```python
from build123d import *

# Parameters (mm, degrees)
SKETCH2_R           = 6
BOSS_EXTRUDE2_DEPTH = 70
CUT_EXTRUDE1_DEPTH  = 21.875
CUT_EXTRUDE3_START  = -21.875
CUT_EXTRUDE3_DEPTH  = 21.875
SKETCH4_R           = 4.215
CUT_EXTRUDE4_DEPTH  = 72.470273541


with BuildPart() as part:
    # Sketch2 → Boss-Extrude2 (new body)
    with BuildSketch(Plane.XY):
        with BuildLine():
            ThreePointArc((-6, 0), (0, 6), (6, 0))
            Line((6, 0), (6, 5.291502622))
            ThreePointArc((6, 5.291502622), (0, 8), (-6, 5.291502622))
            Line((-6, 5.291502622), (-6, 0))
        make_face()
        Circle(SKETCH2_R)
        with BuildLine():
            Line((6, -5.291502622), (6, 0))
            ThreePointArc((6, 0), (0, -6), (-6, 0))
            Line((-6, 0), (-6, -5.291502622))
            ThreePointArc((-6, -5.291502622), (0, -8), (6, -5.291502622))
        make_face()
    extrude(amount=-BOSS_EXTRUDE2_DEPTH)

    # Sketch5 → Cut-Extrude1 (cut)
    with BuildSketch(Plane.XY):
        with BuildLine():
            ThreePointArc((6, 5.291502622), (0, 8), (-6, 5.291502622))
            Line((-6, 5.291502622), (-6, -5e-09))
            ThreePointArc((-6, -5e-09), (-2e-09, 6), (6, 0))
            Line((6, 0), (6, 5.291502622))
        make_face()
        with BuildLine():
            ThreePointArc((6, 0), (2e-09, -6), (-6, -5e-09))
            Line((-6, -5e-09), (-6, -5.291502622))
            ThreePointArc((-6, -5.291502622), (0, -8), (6, -5.291502622))
            Line((6, -5.291502622), (6, 0))
        make_face()
    extrude(amount=-CUT_EXTRUDE1_DEPTH, mode=Mode.SUBTRACT)

    # Sketch6 → Cut-Extrude3 (cut)
    with BuildSketch(Plane(origin=(0, 0, -70), x_dir=(-1, 0, 0), z_dir=(0, 0, -1)).offset(CUT_EXTRUDE3_START)):
        with BuildLine():
            ThreePointArc((6, 5.291502622), (0, 8), (-6, 5.291502622))
            Line((-6, 5.291502622), (-6, -5e-09))
            ThreePointArc((-6, -5e-09), (-2e-09, 6), (6, 0))
            Line((6, 0), (6, 5.291502622))
        make_face()
        with BuildLine():
            ThreePointArc((6, 0), (2e-09, -6), (-6, -5e-09))
            Line((-6, -5e-09), (-6, -5.291502622))
            ThreePointArc((-6, -5.291502622), (0, -8), (6, -5.291502622))
            Line((6, -5.291502622), (6, 0))
        make_face()
    extrude(amount=CUT_EXTRUDE3_DEPTH, mode=Mode.SUBTRACT)

    # Sketch4 → Cut-Extrude4 (cut, through all)
    with BuildSketch(Plane(origin=(6, 0, 0), x_dir=(0, 0, -1), z_dir=(1, 0, 0))):
        with Locations((35, 0)):
            Circle(SKETCH4_R)
    extrude(amount=-CUT_EXTRUDE4_DEPTH, mode=Mode.SUBTRACT)


solid = part.part
```
Input: part model. Units: mm. Frame: model coordinates. A direction names the side the tool comes from. Coordinates: 2 decimals unless noted, no trailing zeros. Write each loop counter-clockwise with the first axis right and the second up, starting at its lowest first coordinate (ties: lowest second). Pieces come first, ordered by that corner, then holes.
1) Pin query (flat end, axial travel): pin 1 Ø5 at (x, z) = (3, -48.5) entering from -Y; pin 2 Ø7.5 at (y, z) = (0, -35) entering from +X; pin 3 Ø1 at (y, z) = (-2.5, -13) entering from +X. Return the tip coordinate at first contact, or that it passes through.
2) Set-up query: faces 1 (the flat face through (0.4, -6.4, -21.875)), 2 (the cylindrical face through (4.76, 3.65, -58.91)), 3 (the flat face through (-0.4, 6.4, -48.125)), 4 (the flat face through (-0.4, -6.4, -48.125)). Return all of +Z, -Z, +X, -X, +Y, -Y with unobstructed straight access to the full face (end or side cutting, diameter ignored); none if empty.
3) Section B-B on x = 0. Output: boundary loops of the cut face in (y, z) (3 decimals).
4) Section A-A on z = -35. Output: boundary loops of the cut face in (x, y) (1 decimal).
5) Section D-D on z = -65. Output: boundary loops of the cut face in (x, y), and give its area (3 significant figures).
6) Mould query, pull axis Y, two halves, no side actions, for faces 5 (the cylindrical face through (0, -8, -35)), 6 (the flat face through (0, 0, 0)), 7 (the cylindrical face through (0.08, 0.19, -30.79)). Classes: pulls with the +Y half, pulls with the -Y half, needs draft (parallel to the pull), parting line crosses it, or undercut.
7) Section C-C on y = 1.25. Output: boundary loops of the cut face in (x, z) (3 decimals), and give its area (3 significant figures).
8) Material intervals for line 1 along Y through (x, z) = (2.25, -35) (3 decimals); line 2 along Y through (x, z) = (2.5, -35) (3 decimals); line 3 along Y through (x, z) = (-0.25, -44), sorted ascending.
Check result:
1. pin 1: stops at y = -7.98
1. pin 2: passes through
1. pin 3: stops at x = 5.66
2. face 1: +Z, -Y
2. face 2: -Z
2. face 3: -Z, +Y
2. face 4: -Z, -Y
3. outline: (-8, -48.125) - (-6, -48.125) - (-6, -70) - (6, -70) - (6, -48.125) - (8, -48.125) - (8, -21.875) - (6, -21.875) - (6, 0) - (-6, 0) - (-6, -21.875) - (-8, -21.875) - close; hole circle Ø8.43 at (0, -35)
4. outline: (-6, -5.3) arc R8 ccw to (6, -5.3) - (6, -4.2) - (-6, -4.2) - close; (-6, 4.2) - (6, 4.2) - (6, 5.3) arc R8 ccw to (-6, 5.3) - close
5. outline: circle Ø12 at (0, 0)
5. area: 113 mm2
6. face 5: pulls with the -Y half
6. face 6: needs draft
6. face 7: undercut
7. outline: (-6, -48.125) - (-5.868, -48.125) - (-5.868, -70) - (5.868, -70) - (5.868, -48.125) - (6, -48.125) - (6, -39.025) - (-6, -39.025) - close; (-6, -30.975) - (6, -30.975) - (6, -21.875) - (5.868, -21.875) - (5.868, 0) - (-5.868, 0) - (-5.868, -21.875) - (-6, -21.875) - close
7. area: 732 mm2
8. line 1: y = -7.677 to -4.215, 4.215 to 7.677
8. line 2: y = -7.599 to -4.215, 4.215 to 7.599
8. line 3: y = -8 to 8
